from build123d import *

# Parameters (mm, degrees)
F1_DEPTH = 60
F3_DEPTH = 8
F4_R     = 0.4
F5_DEPTH = 10
F6_W     = 5
F6_H     = 5
F7_DEPTH = 25


with BuildPart() as f1:
    # F0 (on Right) → F1 (new body)
    with BuildSketch(Plane.YZ):
        with BuildLine():
            ThreePointArc((4.3, 2.8), (3.86066, 3.86066), (2.8, 4.3))
            Line((2.8, 4.3), (-2.8, 4.3))
            ThreePointArc((-2.8, 4.3), (-3.86066, 3.86066), (-4.3, 2.8))
            Line((-4.3, 2.8), (-4.3, -2.8))
            ThreePointArc((-4.3, -2.8), (-3.86066, -3.86066), (-2.8, -4.3))
            Line((-2.8, -4.3), (2.8, -4.3))
            ThreePointArc((2.8, -4.3), (3.86066, -3.86066), (4.3, -2.8))
            Line((4.3, -2.8), (4.3, 2.8))
        make_face()
    extrude(amount=F1_DEPTH)

    # F2 (on face) → F3 (join)
    with BuildSketch(Plane.YZ.offset(60)):
        with BuildLine():
            Line((2.8, 3.5), (-2.8, 3.5))
            ThreePointArc((-2.8, 3.5), (-3.294975, 3.294975), (-3.5, 2.8))
            Line((-3.5, 2.8), (-3.5, -2.8))
            ThreePointArc((-3.5, -2.8), (-3.294975, -3.294975), (-2.8, -3.5))
            Line((-2.8, -3.5), (2.8, -3.5))
            ThreePointArc((2.8, -3.5), (3.294975, -3.294975), (3.5, -2.8))
            Line((3.5, -2.8), (3.5, 2.8))
            ThreePointArc((3.5, 2.8), (3.294975, 3.294975), (2.8, 3.5))
        make_face()
    extrude(amount=F3_DEPTH)

    # F4 (on face) → F5 (join)
    with BuildSketch(Plane(origin=(0, 0, 0), x_dir=(0, -1, 0), z_dir=(-1, 0, 0))):
        with Locations((0, 2)):
            Circle(F4_R)
        with Locations((0, -2)):
            Circle(F4_R)
    extrude(amount=F5_DEPTH)

    # F6 (on face) → F7 (cut)
    with BuildSketch(Plane.YZ.offset(68)):
        Rectangle(F6_W, F6_H)
    extrude(amount=-F7_DEPTH, mode=Mode.SUBTRACT)


solid = f1.part
Verification items for the finished model (mm, model axes). A direction names the side the tool comes from. Give positions to 0.01 mm unless a question says otherwise; leave off trailing zeros. Loops run counter-clockwise (first coordinate to the right, second up) from the corner with the lowest first, then second, coordinate; pieces in that order, holes last.
1) Set-up check for faces 1 (the flat face through (64, -3.5, 0)), 2 (the flat face through (56, 2.5, 0)), 3 (the flat face through (64, 0, 3.5)), 4 (the flat face through (64, 0, -3.5)): record each of +Z, -Z, +X, -X, +Y, -Y from which the full face is reachable in a straight line by a thin tool's end or side.
2) Sectioned sample at A-A, the plane x = 44. Enter the section's corners in (y, z).
3) Depth check by flat-ended pin: pin 1 Ø3 at (x, z) = (62, -0.5) entering from +Y; pin 2 Ø4.5 at (x, z) = (65.5, -0.5) entering from -Y; pin 3 Ø4.5 at (x, y) = (65.5, 0.5) entering from -Z. Enter the tip coordinate at first touch or a pass-through.
4) Draft check along Y on faces 5 (the flat face through (30, 0, 4.3)), 6 (the cylindrical face through (29.58, -3.85, 3.87)), 7 (the flat face through (56, -2.5, 0)), 8 (the flat face through (30, 4.3, 0)). Enter one of: pulls with the +Y half, pulls with the -Y half, needs draft (parallel to the pull), parting line crosses it, or undercut.
5) Thickness scan on line 1 along Z through (x, y) = (62, -1.5); line 2 along Y through (x, z) = (56.5, -2). Record the ranges inside material, lowest first.
6) Sectioned sample at B-B, the plane z = 0.25. Enter the section's corners in (x, y), then the cut area to 3 significant figures.
Answers:
1. face 1: +Z, -Z, +X, -Y
1. face 2: +X
1. face 3: +Z, +X, +Y, -Y
1. face 4: -Z, +X, +Y, -Y
2. outline: (-4.3, -2.8) arc R1.5 ccw to (-2.8, -4.3) - (2.8, -4.3) arc R1.5 ccw to (4.3, -2.8) - (4.3, 2.8) arc R1.5 ccw to (2.8, 4.3) - (-2.8, 4.3) arc R1.5 ccw to (-4.3, 2.8) - close; hole (-2.5, -2.5) - (2.5, -2.5) - (2.5, 2.5) - (-2.5, 2.5) - close
3. pin 1: stops at y = 3.5
3. pin 2: stops at y = -3.5
3. pin 3: stops at z = -3.5
4. face 5: needs draft
4. face 6: pulls with the -Y half
4. face 7: undercut
4. face 8: pulls with the +Y half
5. line 1: z = -3.5 to -2.5, 2.5 to 3.5
5. line 2: y = -4.3 to -2.5, 2.5 to 4.3
6. outline: (0, -4.3) - (60, -4.3) - (60, -3.5) - (68, -3.5) - (68, -2.5) - (43, -2.5) - (43, 2.5) - (68, 2.5) - (68, 3.5) - (60, 3.5) - (60, 4.3) - (0, 4.3) - close
6. area: 447 mm2
